from build123d import *

# Parameters (mm, degrees)
F0_R     = 2
F1_DEPTH = 5


with BuildPart() as f1:
    # F0 (on Top) → F1 (new body)
    with BuildSketch(Plane.XY):
        with BuildLine():
            ThreePointArc((-50, 7), (-57, 0), (-50, -7))
            Line((-50, -7), (-1.875644, -7))
            Line((-1.875644, -7), (39.80127, -31.062178))
            ThreePointArc((39.80127, -31.062178), (49.363448, -28.5), (46.80127, -18.937822))
            Line((46.80127, -18.937822), (3.5, 6.062178))
            ThreePointArc((3.5, 6.062178), (1.811733, 6.761481), (0, 7))
            Line((0, 7), (-50, 7))
        make_face()
        with Locations((43.30127, -25)):
            Circle(F0_R, mode=Mode.SUBTRACT)
        with Locations((-50, 0)):
            Circle(F0_R, mode=Mode.SUBTRACT)
        Circle(F0_R, mode=Mode.SUBTRACT)
    extrude(amount=F1_DEPTH)


solid = f1.part
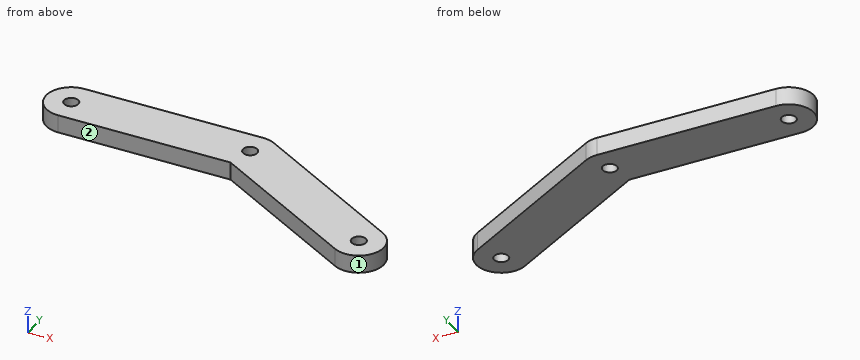
Geometry: final body of the model. Coordinates: model frame, mm. Face numbers are marked on the shaded views. A direction names the side the tool comes from. Give positions to 0.01 mm unless a question says otherwise; leave off trailing zeros. Order: outer loops, then holes, each group sorted by start corner. A loop starts at its lowest first (then second) coordinate and runs counter-clockwise, first axis right, second up. Notation, with made-up numbers: (4, -21.75) -> (58, -21.75) arc R21 ccw to (58, -7.75) -> close; hole circle Ø11 at (-36.75, -11). An arc over 180 degrees is marked (long way). Answer as a JSON object with one key per item and string values.
Q1. First-contact query: pin 1 (1.5 mm diameter, centred on x = 12, z = 1, fed in from -Y). Flat tip, straight axial feed; report the tip coordinate or a pass-through.
Entries:
{"pin 1": "stops at y = -15.44"}
Q2. Section C-C (y = -25). Output: boundary loops of the cut face in (x, z), plus the area to 3 significant figures.
Entries:
{"outline": "(29.3, 0) -> (41.3, 0) -> (41.3, 5) -> (29.3, 5) -> close; (45.3, 0) -> (50.3, 0) -> (50.3, 5) -> (45.3, 5) -> close", "area": "85.0 mm^2"}
Q3. Section D-D (x = -40.5). Output: boundary loops of the cut face in (y, z), plus the area to 3 significant figures.
Entries:
{"outline": "(-7, 0) -> (7, 0) -> (7, 5) -> (-7, 5) -> close", "area": "70.0 mm^2"}
Q4. Material intervals for probe 1 along Y at (x, z) = (-50, 2.4); probe 2 along X at (y, z) = (-1, 3.8); probe 3 along Y at (x, z) = (-23, 1.1), sorted ascending.
Entries:
{"probe 1": "y = -7 to -2, 2 to 7", "probe 2": "x = -56.93 to -51.73, -48.27 to -1.73, 1.73 to 15.73", "probe 3": "y = -7 to 7"}
Q5. Access query for the marked faces 1 and 2. Directions: +Z, -Z, +X, -X, +Y, -Y. A direction counts if a zero-diameter tool reaches every point of the face in a straight line with its end or side. Return the directions, or none.
Entries:
{"face 1": "+Z, -Z", "face 2": "+Z, -Z, -X, -Y"}
Q6. Section A-A (y = 0). Output: boundary loops of the cut face in (x, z), plus the area to 3 significant figures.
Entries:
{"outline": "(-57, 0) -> (-52, 0) -> (-52, 5) -> (-57, 5) -> close; (-48, 0) -> (-2, 0) -> (-2, 5) -> (-48, 5) -> close; (2, 0) -> (14, 0) -> (14, 5) -> (2, 5) -> close", "area": "315 mm^2"}
Q7. Section B-B (z = 3.25). Output: boundary loops of the cut face in (x, y), plus the area to 3 significant figures.
Entries:
{"outline": "(-50, -7) -> (-1.88, -7) -> (39.8, -31.06) arc R7 ccw to (46.8, -18.94) -> (3.5, 6.06) arc R7 ccw to (0, 7) -> (-50, 7) arc R7 ccw to start; hole circle Ø4 at (-50, 0); hole circle Ø4 at (0, 0); hole circle Ø4 at (43.3, -25)", "area": "1,520 mm^2"}
